```python
from build123d import *

# Parameters (mm, degrees)
SKETCH_1_W   = 12
SKETCH_1_H   = 12
SKETCH_1_W_2 = 10
SKETCH_1_H_2 = 10


with BuildPart() as part:
    # 草图1 → ThinRevolve360 (revolve)
    with BuildSketch(Plane.XY, mode=Mode.PRIVATE) as thinrevolve360_sk:
        with Locations((10, 5)):
            Rectangle(SKETCH_1_W, SKETCH_1_H)
        with Locations((10, 5)):
            Rectangle(SKETCH_1_W_2, SKETCH_1_H_2, mode=Mode.SUBTRACT)
    revolve(thinrevolve360_sk.sketch.rotate(Axis((0, 0, 0), (0, 1, 0)), 90), axis=Axis((0, 0, 0), (0, 1, 0)))


solid = part.part
```
Source: CAD feature listing. Evaluate the final solid. Frame: model axes, mm. A direction names the side the tool comes from. Give positions to 0.01 mm unless a question says otherwise; leave off trailing zeros. Write each loop counter-clockwise with the first axis right and the second up, starting at its lowest first coordinate (ties: lowest second). Pieces come first, ordered by that corner, then holes.
1. Material intervals for line 1 along X through (y, z) = (7, 0); line 2 along Y through (x, z) = (0.5, 12.5); line 3 along Z through (x, y) = (-4.5, 2.5), sorted ascending.
2. Section query D-D (z = -12). Return the cut outline in (x, y).
3. Access query for faces 1 (the face through (3.905, 5.084, 0.867)), 2 (the face through (-4, 10, -4)). Directions: +Z, -Z, +X, -X, +Y, -Y. A direction counts if a zero-diameter tool reaches every point of the face in a straight line with its end or side. Return the directions, or none.
4. First-contact query: pin 1 (3 mm diameter, centred on y = 2, z = 2.5, fed in from +X); pin 2 (5 mm diameter, centred on y = 2, z = -9, fed in from -X); pin 3 (1 mm diameter, centred on x = -11.5, y = 1.5, fed in from +Z); pin 4 (18 mm diameter, centred on x = 0, z = 0, fed in from -Y). Flat tips, straight axial feed; report the tip coordinate or a pass-through.
5. Pull-direction query (Z, two-part tool) for faces 3 (the face through (15.62, 5.08, 3.47)), 4 (the face through (-4, 0, -4)), 5 (the face through (3, 11, 3)); classes: +Z half, -Z half, draft (parallel to the pull), parting line (faces both ways), or undercut.
6. Section query B-B (z = 0). Return the cut outline in (x, y), then the cut area to 3 significant figures.
7. Section query A-A (x = 0). Return the cut outline in (y, z).
8. Section query C-C (y = 9). Return the cut outline in (x, z), then the cut area to 3 significant figures.
Output values:
1. line 1: x = -16 to -15, -5 to -4, 4 to 5, 15 to 16
1. line 2: y = -1 to 0, 10 to 11
1. line 3: z = -15.35 to -14.31, -2.18 to 2.18, 14.31 to 15.35
2. outline: (-10.58, -1) - (10.58, -1) - (10.58, 11) - (-10.58, 11) - close; hole (-9, 0) - (9, 0) - (9, 10) - (-9, 10) - close
3. face 1: +Y, -Y
3. face 2: none
4. pin 1: stops at x = 15.97
4. pin 2: stops at x = -14.62
4. pin 3: stops at z = 11.62
4. pin 4: stops at y = -1
5. face 3: parting line
5. face 4: undercut
5. face 5: draft
6. outline: (-16, -1) - (-4, -1) - (-4, 11) - (-16, 11) - close; (4, -1) - (16, -1) - (16, 11) - (4, 11) - close; hole (-15, 0) - (-5, 0) - (-5, 10) - (-15, 10) - close; hole (5, 0) - (15, 0) - (15, 10) - (5, 10) - close
6. area: 88.0 mm2
7. outline: (-1, -16) - (11, -16) - (11, -4) - (-1, -4) - close; (-1, 4) - (11, 4) - (11, 16) - (-1, 16) - close; hole (0, -15) - (10, -15) - (10, -5) - (0, -5) - close; hole (0, 5) - (10, 5) - (10, 15) - (0, 15) - close
8. outline: circle Ø32 at (0, 0); circle Ø10 at (0, 0); hole circle Ø30 at (0, 0); hole circle Ø8 at (0, 0)
8. area: 126 mm2
